```python
from build123d import *

# Parameters (mm, degrees)
SKETCH_1_W          = 42
SKETCH_1_H          = 42
EXTRUDE_1_DEPTH     = 500
SKETCH_2_R          = 11
SKETCH_2_R_2        = 1.5
CUT_EXTRUDE_1_DEPTH = 3
SKETCH_3_R          = 4
CUT_EXTRUDE_2_DEPTH = 3
SKETCH_4_W          = 36
SKETCH_4_H          = 494
CUT_EXTRUDE_3_DEPTH = 504.515640273


with BuildPart() as part:
    # 草图1 → 凸台-拉伸1 (new body)
    with BuildSketch(Plane(origin=(0, 0, 0), x_dir=(1, 0, 0), z_dir=(0, 1, 0))):
        with Locations((21, -21)):
            Rectangle(SKETCH_1_W, SKETCH_1_H)
    extrude(amount=EXTRUDE_1_DEPTH)

    # 草图2 → 切除-拉伸1 (cut)
    with BuildSketch(Plane.XZ):
        with Locations(Location((21, 21, 0), (0, 0, 270))):
            Circle(SKETCH_2_R)
        with Locations(Location((5.5, 5.5, 0), (0, 0, 270))):
            Circle(SKETCH_2_R_2)
        with Locations(Location((5.5, 36.5, 0), (0, 0, 90))):
            Circle(SKETCH_2_R_2)
        with Locations(Location((36.5, 5.5, 0), (0, 0, 90))):
            Circle(SKETCH_2_R_2)
        with Locations(Location((36.5, 36.5, 0), (0, 0, 270))):
            Circle(SKETCH_2_R_2)
    extrude(amount=-CUT_EXTRUDE_1_DEPTH, mode=Mode.SUBTRACT)

    # 草图3 → 切除-拉伸2 (cut)
    with BuildSketch(Plane(origin=(0, 500, 0), x_dir=(1, 0, 0), z_dir=(0, 1, 0))):
        with Locations(Location((21, -21, 0), (0, 0, 270))):
            Circle(SKETCH_3_R)
    extrude(amount=-CUT_EXTRUDE_2_DEPTH, mode=Mode.SUBTRACT)

    # 草图4 → 切除-拉伸3 (cut, through all)
    with BuildSketch(Plane(origin=(0, 0, 0), x_dir=(0, 0, -1), z_dir=(1, 0, 0))):
        with Locations((-21, 250)):
            Rectangle(SKETCH_4_W, SKETCH_4_H)
    extrude(amount=CUT_EXTRUDE_3_DEPTH, mode=Mode.SUBTRACT)


solid = part.part
```
Input: part model. Units: mm. Frame: model coordinates. A direction names the side the tool comes from. Coordinates: 2 decimals unless noted, no trailing zeros. Order: outer loops, then holes, each group sorted by start corner. A loop starts at its lowest first (then second) coordinate and runs counter-clockwise, first axis right, second up. Notation, with made-up numbers: (-8.75, 65) - (39.25, 65) arc R15 ccw to (39.25, 81) - close; hole circle Ø5 at (-30, -7.5). An arc over 180 degrees is marked (long way). Put each result on its own line as item: value.
1. Line query: line 1 along X through (y, z) = (1.9, 36.5); line 2 along Z through (x, y) = (3, 120); line 3 along Y through (x, z) = (26.5, 8.5). Output: solid intervals per line, ascending.
Report:
line 1: x = 0 to 4, 7 to 35, 38 to 42
line 2: z = 0 to 3, 39 to 42
line 3: y = 0 to 3, 497 to 500
2. Reachability of faces 5 (the face through (21, 247, 3)), 6 (the face through (16, 500, 21)) from +Z, -Z, +X, -X, +Y, -Y: full face, straight path, thin tool, end or side. Return the list, or none.
Report:
face 5: +X, -X
face 6: +Z, -Z, +X, -X, +Y
3. Cut plane A-A on y = 216. Return the cut outline in (x, z), then the cut area to 3 significant figures.
Report:
outline: (0, 0) - (42, 0) - (42, 3) - (0, 3) - close; (0, 39) - (42, 39) - (42, 42) - (0, 42) - close
area: 252 mm2
4. Draft query along Z for faces 1 (the face through (11.241, 1.479, 15.924)), 2 (the face through (30, 0, 30)), 3 (the face through (21, 246, 42)), 4 (the face through (20.7, 497, 25.3)). Return one class per face: pulls with the +Z half, pulls with the -Z half, needs draft (parallel to the pull), parting line crosses it, or undercut.
Report:
face 1: undercut
face 2: needs draft
face 3: pulls with the +Z half
face 4: undercut
5. Contact query for a flat-ended pin moving along its axis: pin 1 Ø2.5 at (x, z) = (5.5, 5.5) entering from -Y. Output: stop coordinate, or through.
Report:
pin 1: stops at y = 497
